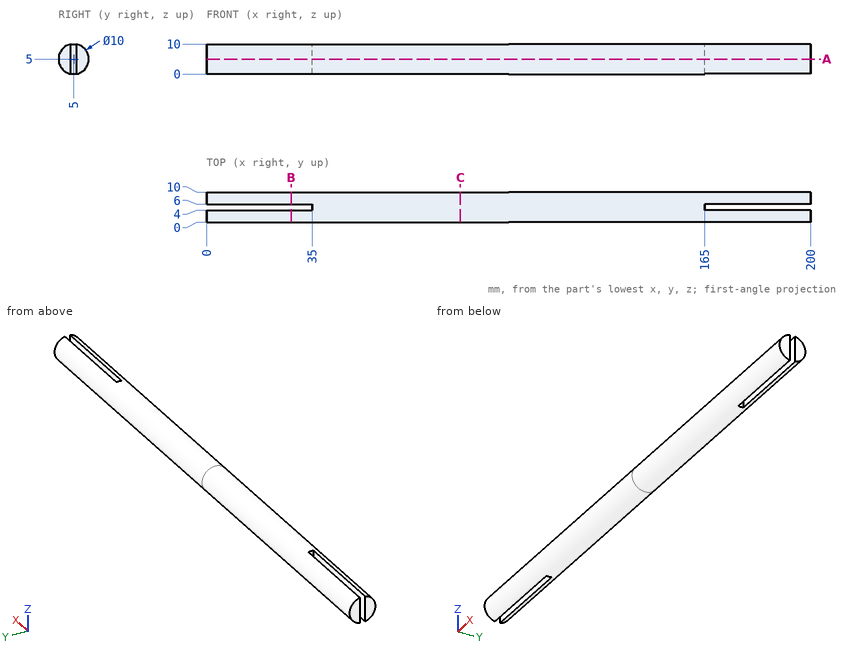
Job drawing, mm, ordinate dimensions from the low corner. One solid piece. Round coordinates to 2 decimals unless told otherwise and drop trailing zeros. Write each loop counter-clockwise with the first axis right and the second up, starting at its lowest first coordinate (ties: lowest second). Pieces come first, ordered by that corner, then holes. Notation, with made-up numbers: (-10, 52.5) -> (49, 52.5) arc R13 cw to (49, 56.5) -> close; hole circle Ø5 at (48, 84.25). An arc over 180 degrees is marked (long way). Answer as a JSON object with one key per item and string values.
(1) Band-saw the part on A-A, the plane z = 5. List the corners of the cut face in (x, y), then the cut area to 3 significant figures.
Reported:
{"outline": "(0, 0) -> (200, 0) -> (200, 4) -> (165, 4) -> (165, 6) -> (200, 6) -> (200, 10) -> (0, 10) -> (0, 6) -> (35, 6) -> (35, 4) -> (0, 4) -> close", "area": "1,860 mm^2"}
(2) Probe probe 1 along X at (y, z) = (5.5, 9.5); probe 2 along Y at (x, z) = (150.5, 4). List the from-to ranges inside material, lowest first. Write a range as [from, to].
Reported:
{"probe 1": "x = [35, 165]", "probe 2": "y = [0.1, 9.9]"}
(3) Band-saw the part on C-C, the plane x = 84. List the corners of the cut face in (y, z), then the cut area to 3 significant figures.
Reported:
{"outline": "circle Ø10 at (5, 5)", "area": "78.5 mm^2"}
(4) Pin check, flat tips, straight feed: P1, Ø0.6, axis at y = 5.5, z = 5, coming from the +X side; P2, Ø2, axis at x = 65.5, y = 6.5, coming from the -Z side; P3, Ø4, axis at x = 172.5, y = 4, coming from the -Z side. Stop position of each tip, or through.
Reported:
{"P1": "stops at x = 165", "P2": "stops at z = 0.03", "P3": "stops at z = 0.1"}
(5) Band-saw the part on B-B, the plane x = 28. List the corners of the cut face in (y, z).
Reported:
{"outline": "(4, 0.1) -> (4, 9.9) arc R5 ccw to start; (6, 0.1) arc R5 ccw to (6, 9.9) -> close"}
